Here's how the part is built. I have some questions about the finished solid (model axes, mm). Face numbers are marked on the shaded views. A direction names the side the tool comes from. Give positions to 0.01 mm unless a question says otherwise; leave off trailing zeros. Loops run counter-clockwise (first coordinate to the right, second up) from the corner with the lowest first, then second, coordinate; pieces in that order, holes last.
Q1. Thinking about a two-plate mould opening in X: for the marked faces 1, 2, 3 and 4, which applies, pulls with the +X half, pulls with the -X half, needs draft (parallel to the pull), parting line crosses it, or undercut?
Q2. Suppose I cut it at C-C (z = -1.1). List the corners of the cut face in (x, y) for me.
Q3. I'm going to push flat-ended pins straight in: P1, Ø3, axis at x = 0, y = 0, coming from the +Z side; P2, Ø2, axis at x = 1, y = 5.5, coming from the -Z side; P3, Ø3, axis at x = -1.5, z = -0.5, coming from the -Y side. Where does each tip first touch, or does it pass through?
Q4. Suppose I cut it at D-D (y = -11). List the corners of the cut face in (x, z) for me, and give its area (4 significant figures).
Q5. Suppose I cut it at B-B (x = 0). Count the separate pieces of the cut face and the enclosed holes in it, and give its area (3 significant figures).
Q6. Suppose I cut it at A-A (y = 5). List the corners of the cut face in (x, z) for me.
Q7. For the marked faces 5 and 6, which set-ups out of +Z, -Z, +X, -X, +Y, -Y let a thin tool reach every point of the face, with its end or its side?
Q8. I need wall thicknesses on probe 1 along Z at (x, y) = (0, 10); probe 2 along Y at (x, z) = (1.5, -2.1); probe 3 along Y at (x, z) = (-1.5, 1.3). Which ranges of each line are inside material? Lowest first, please.
```python
from build123d import *

# Parameters (mm, degrees)
EXTRUDE_1_DEPTH     = 2
SKETCH_2_R          = 3.35
EXTRUDE_2_DEPTH     = 0.3
SKETCH_3_R          = 3.35
EXTRUDE_3_DEPTH     = 2.7
SKETCH_4_R          = 2.45
CUT_EXTRUDE_1_DEPTH = 1.5
SKETCH_5_R          = 1.25
CUT_EXTRUDE_2_DEPTH = 4.5
SKETCH_6_R          = 2.45
CUT_EXTRUDE_3_DEPTH = 3
SKETCH_7_R          = 0.5
CUT_EXTRUDE_4_DEPTH = 5.7


with BuildPart() as part:
    # Эскиз1 → Бобышка-Вытянуть1 (new body)
    with BuildSketch(Plane.XY):
        with BuildLine():
            Line((-3.333438, 0.332705), (-1.890606, 14.788699))
            ThreePointArc((-1.890606, 14.788699), (0, 16.5), (1.890606, 14.788699))
            Line((1.890606, 14.788699), (3.333438, 0.332705))
            ThreePointArc((3.333438, 0.332705), (3.35, 0), (3.333438, -0.332705))
            Line((3.333438, -0.332705), (1.890606, -14.788699))
            ThreePointArc((1.890606, -14.788699), (0, -16.5), (-1.890606, -14.788699))
            Line((-1.890606, -14.788699), (-3.333438, -0.332705))
            ThreePointArc((-3.333438, -0.332705), (-3.35, 0), (-3.333438, 0.332705))
        make_face()
    extrude(amount=EXTRUDE_1_DEPTH)

    # Эскиз2 → Бобышка-Вытянуть2 (add)
    with BuildSketch(Plane.XY.offset(2)):
        Circle(SKETCH_2_R)
    extrude(amount=EXTRUDE_2_DEPTH)

    # Эскиз3 → Бобышка-Вытянуть3 (add)
    with BuildSketch(Plane(origin=(0, 0, 0), x_dir=(-1, 0, 0), z_dir=(0, 0, -1))):
        Circle(SKETCH_3_R)
    extrude(amount=EXTRUDE_3_DEPTH)

    # Эскиз4 → Вырез-Вытянуть1 (cut)
    with BuildSketch(Plane.XY.offset(2.3)):
        Circle(SKETCH_4_R)
    extrude(amount=-CUT_EXTRUDE_1_DEPTH, mode=Mode.SUBTRACT)

    # Эскиз5 → Вырез-Вытянуть2 (cut, through all)
    with BuildSketch(Plane.XY.offset(0.8)):
        Circle(SKETCH_5_R)
    extrude(amount=-CUT_EXTRUDE_2_DEPTH, mode=Mode.SUBTRACT)

    # Эскиз6 → Вырез-Вытянуть3 (cut)
    with BuildSketch(Plane(origin=(0, 0, -2.7), x_dir=(-1, 0, 0), z_dir=(0, 0, -1))):
        Circle(SKETCH_6_R)
    extrude(amount=-CUT_EXTRUDE_3_DEPTH, mode=Mode.SUBTRACT)

    # Эскиз7 → Вырез-Вытянуть4 (cut, through all)
    with BuildSketch(Plane.XY.offset(2)):
        with Locations((0, 15)):
            Circle(SKETCH_7_R)
        with Locations((0, -15)):
            Circle(SKETCH_7_R)
        with Locations((0, -5)):
            Circle(SKETCH_7_R)
        with Locations((0, 5)):
            Circle(SKETCH_7_R)
        with Locations((0, -7)):
            Circle(SKETCH_7_R)
        with Locations((0, 7)):
            Circle(SKETCH_7_R)
        with Locations((0, -9)):
            Circle(SKETCH_7_R)
        with Locations((0, -11)):
            Circle(SKETCH_7_R)
        with Locations((0, 9)):
            Circle(SKETCH_7_R)
        with Locations((0, 11)):
            Circle(SKETCH_7_R)
        with Locations((0, 13)):
            Circle(SKETCH_7_R)
        with Locations((0, -13)):
            Circle(SKETCH_7_R)
    extrude(amount=-CUT_EXTRUDE_4_DEPTH, mode=Mode.SUBTRACT)


solid = part.part
```
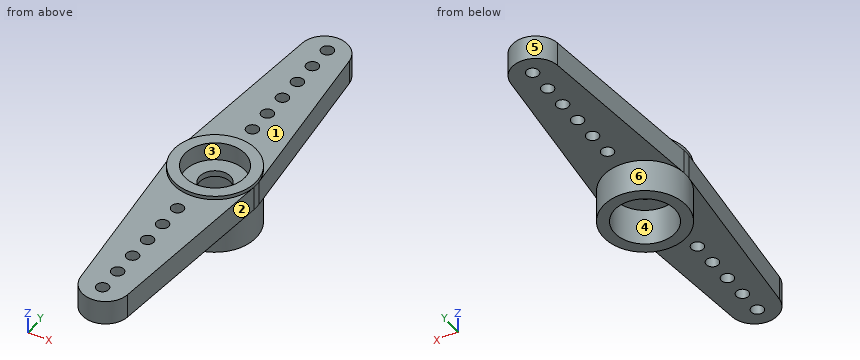
Solutions:
1. face 1: needs draft
1. face 2: pulls with the +X half
1. face 3: undercut
1. face 4: undercut
2. outline: circle Ø6.7 at (0, 0); hole circle Ø4.9 at (0, 0)
3. P1: stops at z = 0.8
3. P2: stops at z = 0
3. P3: stops at y = -16.5
4. outline: (-2.27, 0) - (-0.5, 0) - (-0.5, 2) - (-2.27, 2) - close; (0.5, 0) - (2.27, 0) - (2.27, 2) - (0.5, 2) - close
4. area: 7.075 mm2
5. separate pieces: 14
5. enclosed holes: 0
5. area: 38.8 mm2
6. outline: (-2.87, 0) - (-0.5, 0) - (-0.5, 2) - (-2.87, 2) - close; (0.5, 0) - (2.87, 0) - (2.87, 2) - (0.5, 2) - close
7. face 5: +Z, -Z, +Y
7. face 6: -Z
8. probe 1: z = 0 to 2
8. probe 2: y = -3 to -1.94, 1.94 to 3
8. probe 3: y = -15.77 to -1.94, 1.94 to 15.77
